For this review, take the finished solid that the model builds, in its own axes (mm). A direction names the side the tool comes from. Round coordinates to 2 decimals unless told otherwise and drop trailing zeros. Order: outer loops, then holes, each group sorted by start corner. A loop starts at its lowest first (then second) coordinate and runs counter-clockwise, first axis right, second up. Notation, with made-up numbers: M 75,86.5 L 129,86.5 A7 ccw 129,91.5 Z; hole C 72.25,35 d9. An arc over 180 degrees is marked long. Answer as a JSON object with one key per item and string values.
from build123d import *

# Parameters (mm, degrees)
SKETCH_W        = 31.75
SKETCH_H        = 31.75
SKETCH_W_2      = 26.2128
SKETCH_H_2      = 26.2128
PAD_DEPTH       = 1211.76796
POCKET_DEPTH    = 31.75
POCKET001_DEPTH = 31.75


with BuildPart() as part:
    # Sketch → Pad (new body)
    with BuildSketch(Plane.XZ):
        Rectangle(SKETCH_W, SKETCH_H)
        Rectangle(SKETCH_W_2, SKETCH_H_2, mode=Mode.SUBTRACT)
    extrude(amount=PAD_DEPTH)

    # Sketch001 → Pocket (cut)
    with BuildSketch(Plane(origin=(15.875, 0, 0), x_dir=(0, 0, 1), z_dir=(1, 0, 0))):
        Polygon((15.875, 0), (-15.875, 0), (-15.875, 20.637526), align=None)
    extrude(amount=-POCKET_DEPTH, mode=Mode.SUBTRACT)

    # Sketch002 → Pocket001 (cut)
    with BuildSketch(Plane(origin=(15.875, 0, 0), x_dir=(0, 0, 1), z_dir=(1, 0, 0))):
        Polygon((15.875, 1211.76796), (-15.875, 1211.76796), (-15.875, 1191.130434), align=None)
    extrude(amount=-POCKET001_DEPTH, mode=Mode.SUBTRACT)


solid = part.part
1) Add section A-A on y = -647. State the section outline as (x, z) points (3 decimals), and give its area (3 significant figures).
Geometry check:
{"outline": "M -15.875,-15.875 L 15.875,-15.875 L 15.875,15.875 L -15.875,15.875 Z; hole M -13.106,-13.106 L 13.106,-13.106 L 13.106,13.106 L -13.106,13.106 Z", "area": "321 mm²"}
2) Insertion check: P1, Ø10, axis at x = 1, z = 4, coming from the +Y side. The pin has a flat end and moves straight along its axis. Give the tip position at first contact, or say it passes through.
Geometry check:
{"P1": "passes through"}
3) Add section C-C on z = 3. State the section outline as (x, y) points (3 decimals), and give its area (3 significant figures).
Geometry check:
{"outline": "M -15.875,-1203.399 L -13.106,-1203.399 L -13.106,-8.369 L -15.875,-8.369 Z; M 13.106,-1203.399 L 15.875,-1203.399 L 15.875,-8.369 L 13.106,-8.369 Z", "area": "6,620 mm²"}
4) Add section B-B on x = 3.5. State the section outline as (y, z) points (3 decimals), and give its area (3 significant figures).
Geometry check:
{"outline": "M -1211.768,15.875 L -1209.968,13.106 L -1.8,13.106 L 0,15.875 Z; M -1192.93,-13.106 L -1191.13,-15.875 L -20.638,-15.875 L -18.838,-13.106 Z", "area": "6,600 mm²"}
5) For L1, parallel to Z at x = -5, y = -936.5 (3 decimals); L2, parallel to Y at x = 13.5, z = 11, list the stretches that pass through material, from the lowest coordinate up.
Geometry check:
{"L1": "z = -15.875 to -13.106, 13.106 to 15.875", "L2": "y = -1208.6 to -3.17"}
6) Machinability: for faces 5 (the flat face through (13.106, -597, 0)), 6 (the flat face through (-13.889, -1201.305, -0.222)), which of the approach directions +Z, -Z, +X, -X, +Y, -Y give a long, thin tool a straight path to every point of the face, cutting with its end or side? Answer none if there is none.
Geometry check:
{"face 5": "+Y, -Y", "face 6": "-Z, +X, -X, -Y"}
7) Mouldability with a two-part tool opening along X and no side actions: class faces 1 (the flat face through (-13.89, -10.46, -0.22)), 2 (the flat face through (-13.106, -597, 0)), 3 (the flat face through (-15.875, -597, 0)), 4 (the flat face through (0, -597, 13.106)) as +X half, -X half, draft (parallel to the pull), parting line (faces both ways), or undercut.
Geometry check:
{"face 1": "draft", "face 2": "undercut", "face 3": "-X half", "face 4": "undercut"}
